Design review of the part shown in the three views and the two pictorial views. Dimensions are in mm from the part's minimum x, y and z. A direction names the side the tool comes from. Round coordinates to 2 decimals unless told otherwise and drop trailing zeros. Write each loop counter-clockwise with the first axis right and the second up, starting at its lowest first coordinate (ties: lowest second). Pieces come first, ordered by that corner, then holes. Notation, with made-up numbers: (12.25, 4) -> (42.25, 4) arc R16 cw to (42.25, 29) -> close; hole circle Ø5 at (-2.5, 48). An arc over 180 degrees is marked (long way). One line per question, with ' | ' between items. Start each with the question number.
1) Consider section C-C (x = 40). Give the boundary of the cut face in (y, z).
2) Consider section A-A (z = 5.5). Give the boundary of the cut face in (x, y) (1 decimal).
3) For probe 1 along Z at (x, y) = (53.5, 34); probe 2 along Y at (x, z) = (50, 8.5); probe 3 along X at (y, z) = (27, 17) (1 decimal), list the stretches that pass through material, from the lowest coordinate up.
4) For the marked faces 1, 2 and 3, list the 3-axis set-ups (+Z, -Z, +X, -X, +Y, -Y) from which the entire face can be reached by the end or side of a thin tool; tool diameter is ignored.
5) Consider section D-D (z = 16). Give the boundary of the cut face in (x, y).
6) Insertion check: pin 1 Ø19 at (x, y) = (24.5, 21.5) entering from -Z; pin 2 Ø1.5 at (y, z) = (11.5, 16) entering from -X; pin 3 Ø2.5 at (y, z) = (32, 5) entering from +X (1 decimal); pin 4 Ø5 at (y, z) = (8.5, 17) entering from -X. Each pin has a flat end and moves straight along its axis. Give the tip position at first contact, or say it passes through.
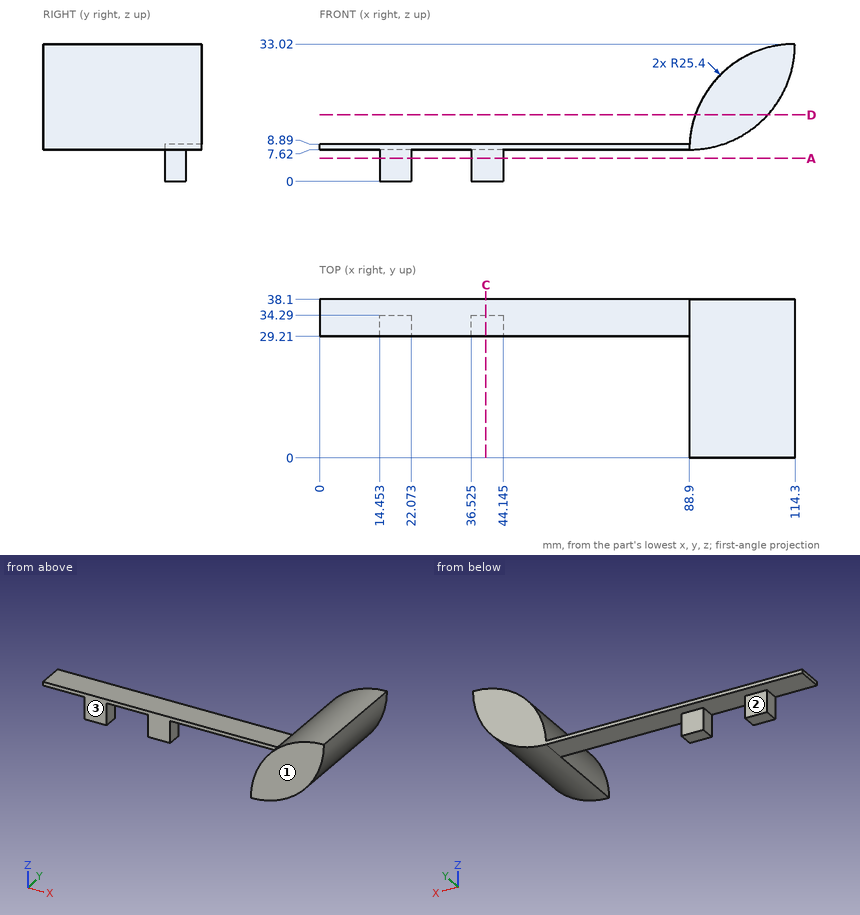
From the geometry:
1) outline: (29.21, 0) -> (34.29, 0) -> (34.29, 7.62) -> (38.1, 7.62) -> (38.1, 8.89) -> (29.21, 8.89) -> close
2) outline: (14.5, 29.2) -> (22.1, 29.2) -> (22.1, 34.3) -> (14.5, 34.3) -> close; (36.5, 29.2) -> (44.1, 29.2) -> (44.1, 34.3) -> (36.5, 34.3) -> close
3) probe 1: z = 7.62 to 8.89 | probe 2: y = 29.21 to 38.1 | probe 3: x = 90.7 to 108.6
4) face 1: +Z, -Z, +X, -X, -Y | face 2: -Z, +X, -X, +Y | face 3: +Z, -Z, -X, -Y
5) outline: (90.32, 0) -> (107.75, 0) -> (107.75, 38.1) -> (90.32, 38.1) -> close
6) pin 1: stops at z = 0 | pin 2: stops at x = 90.07 | pin 3: stops at x = 44.1 | pin 4: stops at x = 89.85
